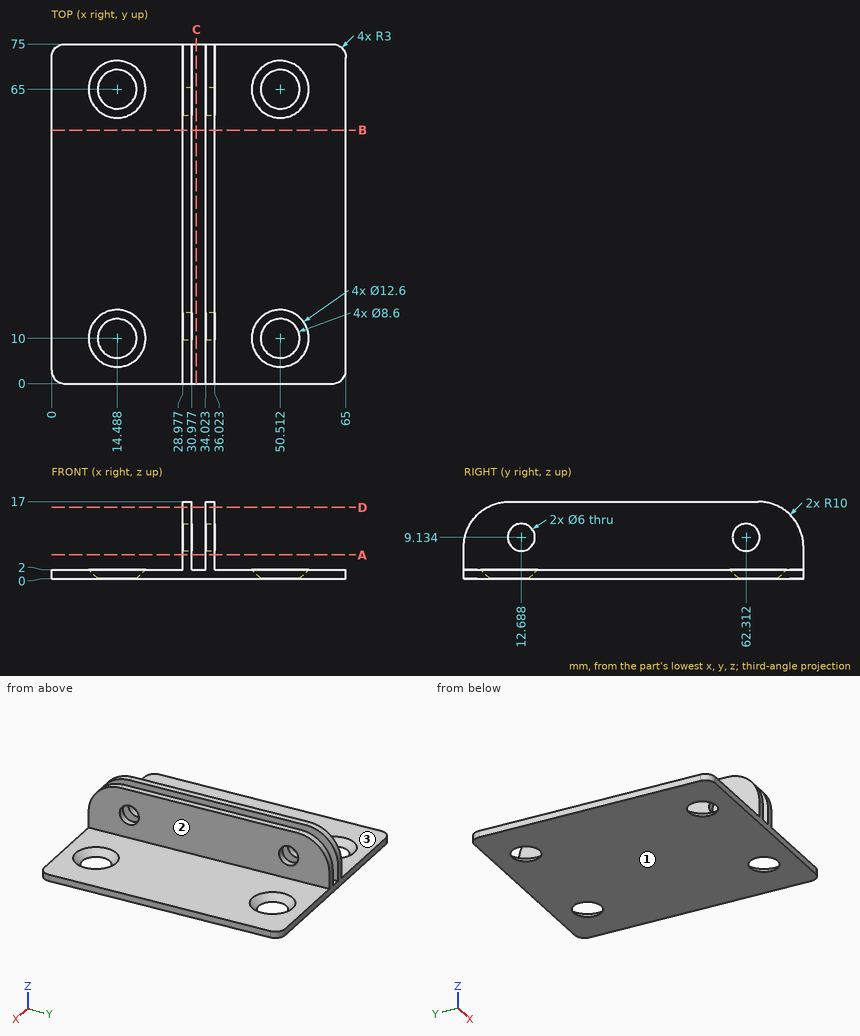
Print and shaded views of the part. All mm, measured from the part's lowest x, y and z. A direction names the side the tool comes from. Give positions to 0.01 mm unless a question says otherwise; leave off trailing zeros. Order: outer loops, then holes, each group sorted by start corner. A loop starts at its lowest first (then second) coordinate and runs counter-clockwise, first axis right, second up. Notation, with made-up numbers: (39, -21) - (54, -21) arc R17 cw to (54, -4) - close; hole circle Ø6 at (-14, 27.5). An arc over 180 degrees is marked (long way). One line per item, written item: value.
Item 1: Tool access for the marked faces 1, 2 and 3: list every direction of +Z, -Z, +X, -X, +Y, -Y with a clear straight run to the whole face (end or side of a thin tool).
Response values:
face 1: -Z, +X, -X, +Y, -Y
face 2: +Z, +X, +Y, -Y
face 3: +Z, -X, +Y, -Y
Item 2: Slice it at C-C (x = 32). List the corners of the cut face in (y, z).
Response values:
outline: (0, 0) - (75, 0) - (75, 2) - (0, 2) - close
Item 3: Slice it at D-D (z = 15.75). List the corners of the cut face in (x, y).
Response values:
outline: (28.98, 5.16) - (30.98, 5.16) - (30.98, 69.84) - (28.98, 69.84) - close; (34.02, 5.16) - (36.02, 5.16) - (36.02, 69.84) - (34.02, 69.84) - close
Item 4: Slice it at A-A (z = 5.25). List the corners of the cut face in (x, y), then the cut area to 3 significant figures.
Response values:
outline: (28.98, 0) - (30.98, 0) - (30.98, 75) - (28.98, 75) - close; (34.02, 0) - (36.02, 0) - (36.02, 75) - (34.02, 75) - close
area: 300 mm2
Item 5: Slice it at B-B (y = 56). List the corners of the cut face in (x, z), then the cut area to 3 significant figures.
Response values:
outline: (0, 0) - (65, 0) - (65, 2) - (36.02, 2) - (36.02, 17) - (34.02, 17) - (34.02, 2) - (30.98, 2) - (30.98, 17) - (28.98, 17) - (28.98, 2) - (0, 2) - close
area: 190 mm2
Item 6: Wall check: line 1 (X direction, y = 63.5, z = 12); line 2 (Z direction, x = 29.5, y = 13); line 3 (Y direction, x = 54, z = 1.75) (1 decimal). Give the ranges that are in metal, low to high.
Response values:
line 1: 28.98 to 30.98, 34.02 to 36.02
line 2: 0 to 6.15, 12.12 to 17
line 3: 0 to 5.1, 14.9 to 60.1, 69.9 to 75
Item 7: Pin check, flat tips, straight feed: pin 1 Ø23 at (x, y) = (13.5, 54.5) entering from +Z; pin 2 Ø2 at (y, z) = (52.5, 9.5) entering from -X; pin 3 Ø4.5 at (y, z) = (46.5, 10.5) entering from +X. Stop position of each tip, or through.
Response values:
pin 1: z = 2
pin 2: x = 28.98
pin 3: x = 36.02
